```python
from build123d import *

# Parameters (mm, degrees)
BOSS_EXTRUDE1_DEPTH     = 7.62
SKETCH5_R               = 15.875
CUT_EXTRUDE2_DEPTH      = 50.8
SKETCH6_R               = 15.875
CUT_EXTRUDE3_DEPTH      = 50.8
CUT_EXTRUDE4_DEPTH      = 1
CUT_EXTRUDE4_DEPTH_BACK = 7.62
CUT_EXTRUDE6_REACH      = 9.62
SKETCH9_R               = 4.826
SKETCH10_W              = 30.48
SKETCH10_H              = 114.3
CUT_EXTRUDE12_DEPTH     = 25.4
CUT_EXTRUDE14_REACH     = 9.62
SKETCH14_R              = 50.8
CUT_EXTRUDE15_REACH     = 9.62
SKETCH15_R              = 50.8
CUT_EXTRUDE17_START     = -7.62
SKETCH18_W              = 300.609514784
SKETCH18_H              = 19.05
CUT_EXTRUDE17_DEPTH     = 7.62
CUT_EXTRUDE18_REACH     = 9.62
SKETCH19_R              = 4.826
CUT_EXTRUDE19_REACH     = 9.62
SKETCH20_W              = 22.86
SKETCH20_H              = 50.8
CUT_EXTRUDE20_REACH     = 9.62
SKETCH21_W              = 12.7
SKETCH21_H              = 95.25


with BuildPart() as part:
    # Sketch2 → Boss-Extrude1 (new body)
    with BuildSketch(Plane.XY):
        Polygon((-189.740054039, 245.383385713), (-375.90852523, -170.414614287), (16.77547477, -170.414614287), (-151.640054039, 245.383385713), align=None)
    extrude(amount=BOSS_EXTRUDE1_DEPTH)

    # Sketch5 → Cut-Extrude2 (cut)
    with BuildSketch(Plane(origin=(0, 0, 0), x_dir=(-1, 0, 0), z_dir=(0, 0, -1))):
        with Locations((375.90852523, -170.414614287)):
            Circle(SKETCH5_R)
    extrude(amount=-CUT_EXTRUDE2_DEPTH, mode=Mode.SUBTRACT)

    # Sketch6 → Cut-Extrude3 (cut)
    with BuildSketch(Plane(origin=(0, 0, 0), x_dir=(-1, 0, 0), z_dir=(0, 0, -1))):
        with Locations((-16.77547477, -170.414614287)):
            Circle(SKETCH6_R)
    extrude(amount=-CUT_EXTRUDE3_DEPTH, mode=Mode.SUBTRACT)

    # Sketch8 → Cut-Extrude4 (cut, two sides)
    with BuildSketch(Plane(origin=(0, 0, 0), x_dir=(-1, 0, 0), z_dir=(0, 0, -1))) as cut_extrude4_sk:
        Polygon((218.448947474, -1130.046710402), (218.448947474, -170.414614287), (218.448947474, -56.114614287), (183.523947474, -56.114614287), (183.523947474, -170.414614287), (183.523947474, -1130.046710402), (183.523947474, -3049.310902633), (218.448947474, -3049.310902633), align=None)
    extrude(amount=CUT_EXTRUDE4_DEPTH, mode=Mode.SUBTRACT)
    extrude(cut_extrude4_sk.sketch, amount=-CUT_EXTRUDE4_DEPTH_BACK, mode=Mode.SUBTRACT)

    # Sketch9 → Cut-Extrude6 (cut, up to next)
    with BuildSketch(Plane(origin=(0, 0, 0), x_dir=(-1, 0, 0), z_dir=(0, 0, -1)), mode=Mode.PRIVATE) as cut_extrude6_sk1:
        with Locations((147.328947474, -122.408614287)):
            Circle(SKETCH9_R)
    cut_extrude6_tool1 = extrude(cut_extrude6_sk1.sketch, amount=-CUT_EXTRUDE6_REACH, mode=Mode.PRIVATE) & part.part
    add(cut_extrude6_tool1.solids().sort_by_distance((-147.328947, -122.408614, 0))[0], mode=Mode.SUBTRACT)
    # Sketch9 → Cut-Extrude6 (cut, up to next)
    with BuildSketch(Plane(origin=(0, 0, 0), x_dir=(-1, 0, 0), z_dir=(0, 0, -1)), mode=Mode.PRIVATE) as cut_extrude6_sk2:
        with Locations((255.278947474, -122.408614287)):
            Circle(SKETCH9_R)
    cut_extrude6_tool2 = extrude(cut_extrude6_sk2.sketch, amount=-CUT_EXTRUDE6_REACH, mode=Mode.PRIVATE) & part.part
    add(cut_extrude6_tool2.solids().sort_by_distance((-255.278947, -122.408614, 0))[0], mode=Mode.SUBTRACT)

    # Sketch10 → Cut-Extrude12 (cut)
    with BuildSketch(Plane(origin=(0, 0, 0), x_dir=(-1, 0, 0), z_dir=(0, 0, -1))):
        with Locations((80.066257047, -113.264614287)):
            Rectangle(SKETCH10_W, SKETCH10_H)
    extrude(amount=-CUT_EXTRUDE12_DEPTH, mode=Mode.SUBTRACT)

    # Sketch14 → Cut-Extrude14 (cut, up to next)
    with BuildSketch(Plane(origin=(0, 0, 0), x_dir=(-1, 0, 0), z_dir=(0, 0, -1)), mode=Mode.PRIVATE) as cut_extrude14_sk1:
        with Locations((-16.77547477, -170.414614287)):
            Circle(SKETCH14_R)
    cut_extrude14_tool1 = extrude(cut_extrude14_sk1.sketch, amount=-CUT_EXTRUDE14_REACH, mode=Mode.PRIVATE) & part.part
    add(cut_extrude14_tool1.solids().sort_by_distance((16.775475, -170.414614, 0))[0], mode=Mode.SUBTRACT)

    # Sketch15 → Cut-Extrude15 (cut, up to next)
    with BuildSketch(Plane(origin=(0, 0, 0), x_dir=(-1, 0, 0), z_dir=(0, 0, -1)), mode=Mode.PRIVATE) as cut_extrude15_sk1:
        with Locations((375.90852523, -170.414614287)):
            Circle(SKETCH15_R)
    cut_extrude15_tool1 = extrude(cut_extrude15_sk1.sketch, amount=-CUT_EXTRUDE15_REACH, mode=Mode.PRIVATE) & part.part
    add(cut_extrude15_tool1.solids().sort_by_distance((-375.908525, -170.414614, 0))[0], mode=Mode.SUBTRACT)

    # Sketch18 → Cut-Extrude17 (cut)
    with BuildSketch(Plane(origin=(0, 0, 0), x_dir=(-1, 0, 0), z_dir=(0, 0, -1)).offset(CUT_EXTRUDE17_START)):
        with Locations((180.749872138, -160.889614287)):
            Rectangle(SKETCH18_W, SKETCH18_H)
    extrude(amount=CUT_EXTRUDE17_DEPTH, mode=Mode.SUBTRACT)

    # Sketch19 → Cut-Extrude18 (cut, up to next)
    with BuildSketch(Plane(origin=(0, 0, 0), x_dir=(-1, 0, 0), z_dir=(0, 0, -1)), mode=Mode.PRIVATE) as cut_extrude18_sk1:
        with Locations((255.278947474, -46.208614287)):
            Circle(SKETCH19_R)
    cut_extrude18_tool1 = extrude(cut_extrude18_sk1.sketch, amount=-CUT_EXTRUDE18_REACH, mode=Mode.PRIVATE) & part.part
    add(cut_extrude18_tool1.solids().sort_by_distance((-255.278947, -46.208614, 0))[0], mode=Mode.SUBTRACT)
    # Sketch19 → Cut-Extrude18 (cut, up to next)
    with BuildSketch(Plane(origin=(0, 0, 0), x_dir=(-1, 0, 0), z_dir=(0, 0, -1)), mode=Mode.PRIVATE) as cut_extrude18_sk2:
        with Locations((147.328947474, -46.208614287)):
            Circle(SKETCH19_R)
    cut_extrude18_tool2 = extrude(cut_extrude18_sk2.sketch, amount=-CUT_EXTRUDE18_REACH, mode=Mode.PRIVATE) & part.part
    add(cut_extrude18_tool2.solids().sort_by_distance((-147.328947, -46.208614, 0))[0], mode=Mode.SUBTRACT)

    # Sketch20 → Cut-Extrude19 (cut, up to next)
    with BuildSketch(Plane(origin=(0, 0, 0), x_dir=(-1, 0, 0), z_dir=(0, 0, -1)), mode=Mode.PRIVATE) as cut_extrude19_sk1:
        with Locations((168.664947474, -10.934247938)):
            Rectangle(SKETCH20_W, SKETCH20_H)
    cut_extrude19_tool1 = extrude(cut_extrude19_sk1.sketch, amount=-CUT_EXTRUDE19_REACH, mode=Mode.PRIVATE) & part.part
    add(cut_extrude19_tool1.solids().sort_by_distance((-168.664947, -10.934248, 0))[0], mode=Mode.SUBTRACT)
    # Sketch20 → Cut-Extrude19 (cut, up to next)
    with BuildSketch(Plane(origin=(0, 0, 0), x_dir=(-1, 0, 0), z_dir=(0, 0, -1)), mode=Mode.PRIVATE) as cut_extrude19_sk2:
        with Locations((233.942947474, -10.934247938)):
            Rectangle(SKETCH20_W, SKETCH20_H)
    cut_extrude19_tool2 = extrude(cut_extrude19_sk2.sketch, amount=-CUT_EXTRUDE19_REACH, mode=Mode.PRIVATE) & part.part
    add(cut_extrude19_tool2.solids().sort_by_distance((-233.942947, -10.934248, 0))[0], mode=Mode.SUBTRACT)

    # Sketch21 → Cut-Extrude20 (cut, up to next)
    with BuildSketch(Plane(origin=(0, 0, 0), x_dir=(-1, 0, 0), z_dir=(0, 0, -1)), mode=Mode.PRIVATE) as cut_extrude20_sk1:
        with Locations((224.798947474, -103.739614287)):
            Rectangle(SKETCH21_W, SKETCH21_H)
    cut_extrude20_tool1 = extrude(cut_extrude20_sk1.sketch, amount=-CUT_EXTRUDE20_REACH, mode=Mode.PRIVATE) & part.part
    add(cut_extrude20_tool1.solids().sort_by_distance((-224.798947, -103.739614, 0))[0], mode=Mode.SUBTRACT)
    # Sketch21 → Cut-Extrude20 (cut, up to next)
    with BuildSketch(Plane(origin=(0, 0, 0), x_dir=(-1, 0, 0), z_dir=(0, 0, -1)), mode=Mode.PRIVATE) as cut_extrude20_sk2:
        with Locations((177.173947474, -103.739614287)):
            Rectangle(SKETCH21_W, SKETCH21_H)
    cut_extrude20_tool2 = extrude(cut_extrude20_sk2.sketch, amount=-CUT_EXTRUDE20_REACH, mode=Mode.PRIVATE) & part.part
    add(cut_extrude20_tool2.solids().sort_by_distance((-177.173947, -103.739614, 0))[0], mode=Mode.SUBTRACT)


solid = part.part
```
Part model, mm, in its own coordinate system. Coordinates: 2 decimals unless noted, no trailing zeros. Write each loop counter-clockwise with the first axis right and the second up, starting at its lowest first coordinate (ties: lowest second). Pieces come first, ordered by that corner, then holes.
Item 1: Slice it at B-B (z = 5). Write the cut outline in (x, y), and give its area (3 significant figures).
Item 2: Slice it at C-C (x = -294). Write the cut outline in (y, z), and give its area (3 significant figures).
Item 3: Probe line 1 (Y direction, x = -147.5, z = 2.5); line 2 (X direction, y = -111.5, z = 3.5); line 3 (X direction, y = -66.5, z = 4). List the from-to ranges inside material, lowest first.
Item 4: Pin check, flat tips, straight feed: pin 1 (8.5 mm diameter, centred on x = -147.33, y = -46.21, fed in from -Z); pin 2 (1.5 mm diameter, centred on y = 23, z = 4, fed in from +X); pin 3 (2.5 mm diameter, centred on x = -238, z = 3, fed in from +Y); pin 4 (2.5 mm diameter, centred on y = -9.5, z = 2.5, fed in from -X). Stop position of each tip, or through.
Item 5: Slice it at A-A (y = 3.5). Write the cut outline in (x, z), and give its area (3 significant figures).
Item 6: Mould opens along Y. For faces 1 (the face through (-271.29, 63.25, 3.76)), 2 (the face through (-259.882, -44.759, 3.757)), 3 (the face through (-181, 6, 0)), 4 (the face through (-339.526, -134.961, 3.757)) say: released by +Y, released by -Y, zero draft, split by the parting line, or undercut.
Item 7: Slice it at D-D (y = 152). Write the cut outline in (x, z).
Results found:
1. outline: (-355.15, -124.05) arc R50.8 cw to (-328.82, -151.36) - (-231.15, -151.36) - (-231.15, -56.11) - (-170.82, -56.11) - (-170.82, -151.36) - (-95.31, -151.36) - (-95.31, -56.11) - (-64.83, -56.11) - (-64.83, -151.36) - (-30.45, -151.36) - (-30.45, -151.68) arc R50.8 cw to (-2.3, -123.33) - (-151.64, 245.38) - (-189.74, 245.38) - close; hole circle Ø9.65 at (-255.28, -122.41); hole circle Ø9.65 at (-255.28, -46.21); hole (-245.37, -36.33) - (-222.51, -36.33) - (-222.51, 14.47) - (-245.37, 14.47) - close; hole (-180.09, -36.33) - (-157.23, -36.33) - (-157.23, 14.47) - (-180.09, 14.47) - close; hole circle Ø9.65 at (-147.33, -122.41); hole circle Ø9.65 at (-147.33, -46.21)
1. area: 69,700 mm2
2. outline: (-151.36, 0) - (12.52, 0) - (12.52, 7.62) - (-151.36, 7.62) - close
2. area: 1,250 mm2
3. line 1: y = -151.36 to -127.23, -117.59 to -51.03, -41.39 to 235.16
3. line 2: x = -349.53 to -231.15, -170.82 to -95.31, -64.83 to -7.09
3. line 3: x = -329.38 to -231.15, -170.82 to -95.31, -64.83 to -25.31
4. pin 1: passes through
4. pin 2: stops at x = -61.26
4. pin 3: stops at y = 140.39
4. pin 4: stops at x = -304.42
5. outline: (-298.04, 0) - (-245.37, 0) - (-245.37, 7.62) - (-298.04, 7.62) - close; (-222.51, 0) - (-180.09, 0) - (-180.09, 7.62) - (-222.51, 7.62) - close; (-157.23, 0) - (-53.67, 0) - (-53.67, 7.62) - (-157.23, 7.62) - close
5. area: 1,510 mm2
6. face 1: released by +Y
6. face 2: undercut
6. face 3: zero draft
6. face 4: released by -Y
7. outline: (-231.55, 0) - (-113.82, 0) - (-113.82, 7.62) - (-231.55, 7.62) - close
